```python
from build123d import *

# Parameters (mm, degrees)
SKETCH_1_R      = 1.65
EXTRUDE_1_DEPTH = 2
FILLET_1_R      = 10


with BuildPart() as part:
    # 草图1 → 凸台-拉伸1 (new body)
    with BuildSketch(Plane.XY):
        Polygon((10, 10), (52.276412277, 10), (52.276412277, -10), (-10, -10), (-10, 10), (-10, 50), (10, 50), align=None)
        with Locations((20, 0)):
            Circle(SKETCH_1_R, mode=Mode.SUBTRACT)
        with Locations((3.0503e-05, 20)):
            Circle(SKETCH_1_R, mode=Mode.SUBTRACT)
        with Locations((3.0503e-05, 40)):
            Circle(SKETCH_1_R, mode=Mode.SUBTRACT)
        with Locations((3.0503e-05, 30)):
            Circle(SKETCH_1_R, mode=Mode.SUBTRACT)
        Circle(SKETCH_1_R, mode=Mode.SUBTRACT)
        with Locations((40, 0)):
            Circle(SKETCH_1_R, mode=Mode.SUBTRACT)
    extrude(amount=EXTRUDE_1_DEPTH)

    # 圆角1
    fillet_1_edges = [part.edges().sort_by_distance(p)[0] for p in [
        (10, 10, 1),
    ]]
    fillet(fillet_1_edges, radius=FILLET_1_R)


solid = part.part
```
Part model, mm, in its own coordinate system. A direction names the side the tool comes from. Round coordinates to 2 decimals unless told otherwise and drop trailing zeros. Order: outer loops, then holes, each group sorted by start corner. A loop starts at its lowest first (then second) coordinate and runs counter-clockwise, first axis right, second up. Notation, with made-up numbers: M -17.75,20 L 41.25,20 A21 ccw 41.25,52 Z; hole C 36,-8 d7. An arc over 180 degrees is marked long. Put each result on its own line as item: value. Start each with the question number.
1. Two-plate mould, pull along X, no slides. Class faces 3 (the face through (36, 10, 1)), 4 (the face through (-10, 20, 1)), 5 (the face through (-1.216, 1.115, 0.986)): +X half, -X half, draft (parallel to the pull), parting line (faces both ways), or undercut.
2. Tool access for faces 1 (the face through (-0.215, 31.636, 0.986)), 2 (the face through (10, 35, 1)): list every direction of +Z, -Z, +X, -X, +Y, -Y with a clear straight run to the whole face (end or side of a thin tool).
3. Drill centre lines: probe 1 along Y at (x, z) = (0, 0.55); probe 2 along Y at (x, z) = (20, 1.1); probe 3 along X at (y, z) = (22.5, 1.25). Where is each one in solid material? Low to high. Write a range as [from, to].
4. Slice it at D-D on z = 0.9. List the corners of the cut face in (x, y), then the cut area to 3 significant figures.
5. Slice it at A-A on x = 40. List the corners of the cut face in (y, z).
6. Slice it at C-C on x = 0. List the corners of the cut face in (y, z), then the cut area to 3 significant figures.
Findings:
1. face 3: draft
1. face 4: -X half
1. face 5: undercut
2. face 1: +Z, -Z
2. face 2: +Z, -Z, +X, +Y
3. probe 1: [-10, -1.65], [1.65, 18.35], [21.65, 28.35], [31.65, 38.35], [41.65, 50]
3. probe 2: [-10, -1.65], [1.65, 10]
3. probe 3: [-10, 10]
4. outline: M -10,-10 L 52.28,-10 L 52.28,10 L 20,10 A10 cw 10,20 L 10,50 L -10,50 Z; hole C 0,0 d3.3; hole C 0,20 d3.3; hole C 0,30 d3.3; hole C 0,40 d3.3; hole C 20,0 d3.3; hole C 40,0 d3.3
4. area: 2,020 mm2
5. outline: M -10,0 L -1.65,0 L -1.65,2 L -10,2 Z; M 1.65,0 L 10,0 L 10,2 L 1.65,2 Z
6. outline: M -10,0 L -1.65,0 L -1.65,2 L -10,2 Z; M 1.65,0 L 18.35,0 L 18.35,2 L 1.65,2 Z; M 21.65,0 L 28.35,0 L 28.35,2 L 21.65,2 Z; M 31.65,0 L 38.35,0 L 38.35,2 L 31.65,2 Z; M 41.65,0 L 50,0 L 50,2 L 41.65,2 Z
6. area: 93.6 mm2
